For this review, take the finished solid that the model builds, in its own axes (mm). A direction names the side the tool comes from. Give positions to 0.01 mm unless a question says otherwise; leave off trailing zeros. Loops run counter-clockwise (first coordinate to the right, second up) from the corner with the lowest first, then second, coordinate; pieces in that order, holes last. Notation, with made-up numbers: (39.5, -9.5) - (80.5, -9.5) arc R35 cw to (80.5, 26.5) - close; hole circle Ø1 at (78.5, -3.75). An arc over 180 degrees is marked (long way). Use CSV: the item, a comma, the result in double quotes. Start each with the question number.
1. For faces 4 (the flat face through (-24.562, 3.24, 24.794)), 5 (the flat face through (-16, 2.5, -7)), 6 (the cylindrical face through (-12.583, 1.972, -69.655)), list the 3-axis set-ups (+Z, -Z, +X, -X, +Y, -Y) from which the entire face can be reached by the end or side of a thin tool; tool diameter is ignored.
2. Take a section at A-A on x = 2.5. Give the boundary of the cut face in (y, z).
3. Take a section at D-D on z = -73. Give the boundary of the cut face in (x, y), plus the area to 3 significant figures.
4. Mouldability with a two-part tool opening along Z and no side actions: class faces 1 (the flat face through (-20.09, 3.24, -69.17)), 2 (the flat face through (-19.987, 3.24, 69.48)), 3 (the flat face through (13.265, 2, 0)) as pulls with the +Z half, pulls with the -Z half, needs draft (parallel to the pull), parting line crosses it, or undercut.
5. Wall thickness on line 1 (Z direction, x = 0.5, y = 3.1); line 2 (Z direction, x = -1.5, y = 1.05); line 3 (X direction, y = 0.75, z = -69): over which ranges is each line inside the solid? List them lowest first.
6. For pin 1 (0.8 mm diameter, centred on y = 3, z = -50.5, fed in from -X); pin 2 (1.2 mm diameter, centred on y = 1, z = 2, fed in from +X); pin 3 (1.5 mm diameter, centred on y = 1.5, z = -12.5, fed in from -X); pin 4 (2 mm diameter, centred on x = -1, z = 65, fed in from +Y), all flat-tipped, find the tip position at first contact; note any pin that passes through.
7. Take a section at C-C on z = -41. Give the boundary of the cut face in (x, y), plus the area to 3 significant figures.
```python
from build123d import *

# Parameters (mm, degrees)
BOSS_EXTRUDE1_DEPTH = 2.5
BOSS_EXTRUDE3_DEPTH = 1.5


# Read off the part's stored shape, not the designer's step: Boss-Extrude1
with BuildPart() as part:
    # Boss-Extrude1 outline → Boss-Extrude1 (new body)
    with BuildSketch(Plane(origin=(0, 0, 0), x_dir=(1, 0, 0), z_dir=(0, 1, 0))):
        with BuildLine():
            ThreePointArc((17.600819084, 64.048530094), (13.028302904, 70.558621532), (5.345717729, 68.492930418))
            Line((5.345717729, 68.492930418), (-5.345717729, 68.492930418))
            ThreePointArc((-5.345717729, 68.492930418), (-13.028302904, 70.558621532), (-17.600819084, 64.048530094))
            Line((-17.600819084, 64.048530094), (-17.600819084, 27.344801488))
            Line((-17.600819084, 27.344801488), (-14.264554689, 22.498047837))
            Line((-14.264554689, 22.498047837), (-14.264554689, -22.498047837))
            Line((-14.264554689, -22.498047837), (-17.600819084, -27.344801488))
            Line((-17.600819084, -27.344801488), (-17.600819084, -64.048530094))
            ThreePointArc((-17.600819084, -64.048530094), (-13.028302904, -70.558621532), (-5.345717729, -68.492930418))
            Line((-5.345717729, -68.492930418), (5.345717729, -68.492930418))
            ThreePointArc((5.345717729, -68.492930418), (13.028302904, -70.558621532), (17.600819084, -64.048530094))
            Line((17.600819084, -64.048530094), (17.600819084, -27.344801488))
            Line((17.600819084, -27.344801488), (14.264554689, -22.498047837))
            Line((14.264554689, -22.498047837), (14.264554689, 22.498047837))
            Line((14.264554689, 22.498047837), (17.600819084, 27.344801488))
            Line((17.600819084, 27.344801488), (17.600819084, 64.048530094))
        make_face()
        with BuildLine():
            Line((16.600819084, -27.655707745), (16.600819084, -64.025237528))
            ThreePointArc((16.600819084, -64.025237528), (12.483449957, -69.688325839), (5.834875923, -67.492930418))
            Line((5.834875923, -67.492930418), (-5.834875923, -67.492930418))
            ThreePointArc((-5.834875923, -67.492930418), (-12.483449957, -69.688325839), (-16.600819084, -64.025237528))
            Line((-16.600819084, -64.025237528), (-16.600819084, -27.655707745))
            Line((-16.600819084, -27.655707745), (-13.264554689, -22.808954094))
            Line((-13.264554689, -22.808954094), (-13.264554689, 22.808954094))
            Line((-13.264554689, 22.808954094), (-16.600819084, 27.655707745))
            Line((-16.600819084, 27.655707745), (-16.600819084, 64.025237528))
            ThreePointArc((-16.600819084, 64.025237528), (-12.483449957, 69.688325839), (-5.834875923, 67.492930418))
            Line((-5.834875923, 67.492930418), (5.834875923, 67.492930418))
            ThreePointArc((5.834875923, 67.492930418), (12.483449957, 69.688325839), (16.600819084, 64.025237528))
            Line((16.600819084, 64.025237528), (16.600819084, 27.655707745))
            Line((16.600819084, 27.655707745), (13.264554689, 22.808954094))
            Line((13.264554689, 22.808954094), (13.264554689, -22.808954094))
            Line((13.264554689, -22.808954094), (16.600819084, -27.655707745))
        make_face(mode=Mode.SUBTRACT)
    extrude(amount=BOSS_EXTRUDE1_DEPTH)

    # Sketch4 → Boss-Extrude3 (add)
    with BuildSketch(Plane(origin=(0, 2.5, 0), x_dir=(1, 0, 0), z_dir=(0, 1, 0))):
        Polygon((-9.982037134, 86.769350006), (9.982037134, 86.769350006), (16.264456892, 80.486930248), (23.81578312, 58.16008483), (23.81578312, 47.812822946), (21.672882272, 47.812822946), (21.672882272, 27.300144084), (27.53346101, 22.216178317), (27.53346101, 15.033319747), (23.968939697, 10.924291721), (23.968939697, -10.924291721), (27.53346101, -15.033319747), (27.53346101, -22.216178317), (21.672882272, -27.300144084), (21.672882272, -47.812822946), (23.81578312, -47.812822946), (23.81578312, -58.16008483), (16.264456892, -80.486930248), (9.982037134, -86.769350006), (-9.982037134, -86.769350006), (-16.264456892, -80.486930248), (-23.81578312, -58.16008483), (-23.81578312, -47.812822946), (-21.672882272, -47.812822946), (-21.672882272, -27.300144084), (-27.53346101, -22.216178317), (-27.53346101, -15.033319747), (-23.968939697, -10.924291721), (-23.968939697, 10.924291721), (-27.53346101, 15.033319747), (-27.53346101, 22.216178317), (-21.672882272, 27.300144084), (-21.672882272, 47.812822946), (-23.81578312, 47.812822946), (-23.81578312, 58.16008483), (-16.264456892, 80.486930248), align=None)
        with BuildLine():
            Line((13.264554689, 22.808954094), (13.264554689, -22.808954094))
            Line((13.264554689, -22.808954094), (16.600819084, -27.655707745))
            Line((16.600819084, -27.655707745), (16.600819084, -64.025237528))
            ThreePointArc((16.600819084, -64.025237528), (12.483449957, -69.688325839), (5.834875923, -67.492930418))
            Line((5.834875923, -67.492930418), (-5.834875923, -67.492930418))
            ThreePointArc((-5.834875923, -67.492930418), (-12.483449957, -69.688325839), (-16.600819084, -64.025237528))
            Line((-16.600819084, -64.025237528), (-16.600819084, -27.655707745))
            Line((-16.600819084, -27.655707745), (-13.264554689, -22.808954094))
            Line((-13.264554689, -22.808954094), (-13.264554689, 22.808954094))
            Line((-13.264554689, 22.808954094), (-16.600819084, 27.655707745))
            Line((-16.600819084, 27.655707745), (-16.600819084, 64.025237528))
            ThreePointArc((-16.600819084, 64.025237528), (-12.483449957, 69.688325839), (-5.834875923, 67.492930418))
            Line((-5.834875923, 67.492930418), (5.834875923, 67.492930418))
            ThreePointArc((5.834875923, 67.492930418), (12.483449957, 69.688325839), (16.600819084, 64.025237528))
            Line((16.600819084, 64.025237528), (16.600819084, 27.655707745))
            Line((16.600819084, 27.655707745), (13.264554689, 22.808954094))
        make_face(mode=Mode.SUBTRACT)
    extrude(amount=BOSS_EXTRUDE3_DEPTH)


solid = part.part
```
Check result:
1,face 4,"-X, +Y, -Y"
1,face 5,"-Y"
1,face 6,"+Y, -Y"
2,outline,"(0, -68.49) - (2.5, -68.49) - (2.5, -86.77) - (4, -86.77) - (4, -67.49) - (0, -67.49) - close; (0, 67.49) - (4, 67.49) - (4, 86.77) - (2.5, 86.77) - (2.5, 68.49) - (0, 68.49) - close"
3,outline,"(-18.8, 2.5) - (18.8, 2.5) - (18.8, 4) - (-18.8, 4) - close"
3,area,"56.4 mm²"
4,face 1,"pulls with the -Z half"
4,face 2,"pulls with the +Z half"
4,face 3,"undercut"
5,line 1,"z = -86.77 to -67.49, 67.49 to 86.77"
5,line 2,"z = -68.49 to -67.49, 67.49 to 68.49"
5,line 3,"x = -15.51 to -13.92, -7.4 to -5.82, 5.82 to 7.4, 13.92 to 15.51"
6,pin 1,"stops at x = -23.82"
6,pin 2,"stops at x = 14.26"
6,pin 3,"stops at x = -14.26"
6,pin 4,"passes through"
7,outline,"(-21.67, 2.5) - (-17.6, 2.5) - (-17.6, 0) - (-16.6, 0) - (-16.6, 4) - (-21.67, 4) - close; (16.6, 0) - (17.6, 0) - (17.6, 2.5) - (21.67, 2.5) - (21.67, 4) - (16.6, 4) - close"
7,area,"20.2 mm²"
